Design review of the part shown in the three views and the two pictorial views. Dimensions are in mm from the part's minimum x, y and z. Round coordinates to 2 decimals unless told otherwise and drop trailing zeros. Loops run counter-clockwise (first coordinate to the right, second up) from the corner with the lowest first, then second, coordinate; pieces in that order, holes last. Notation, with made-up numbers: (9, 63) -> (35, 63) arc R26 cw to (35, 90) -> close; hole circle Ø10 at (60, 70). An arc over 180 degrees is marked (long way). Use a Markdown table: item, result. Add a question column.
1) Consider section B-B on x = 33. Give the boundary of the cut face in (y, z).
2) Consider section C-C on y = 2.4. Give the boundary of the cut face in (x, z), plus the area to 3 significant figures.
3) Wall thickness on probe 1 along Y at (x, z) = (79, 32); probe 2 along X at (y, z) = (0.9, 31.5); probe 3 along Z at (x, y) = (35, 3.2): over which ranges is each line inside the solid? List them lowest first.
4) Insertion check: pin 1 (1.6 mm diameter, centred on x = 32.5, y = 2.5, fed in from -Z); pin 2 (1.6 mm diameter, centred on x = 42.5, z = 34.5, fed in from -Y); pin 3 (3 mm diameter, centred on y = 4, z = 6.5, fed in from -X). Each pin has a flat end and moves straight along its axis. Give the tip position at first contact, or say it passes through.
5) Consider section A-A on z = 30. Give the boundary of the cut face in (x, y), plus the area to 3 significant figures.
6) Mouldability with a two-part tool opening along Y and no side actions: class the marked faces 1, 2 and 3 as released by +Y, released by -Y, zero draft, split by the parting line, or undercut.
7) Consider section D-D on z = 5. Give the boundary of the cut face in (x, y).
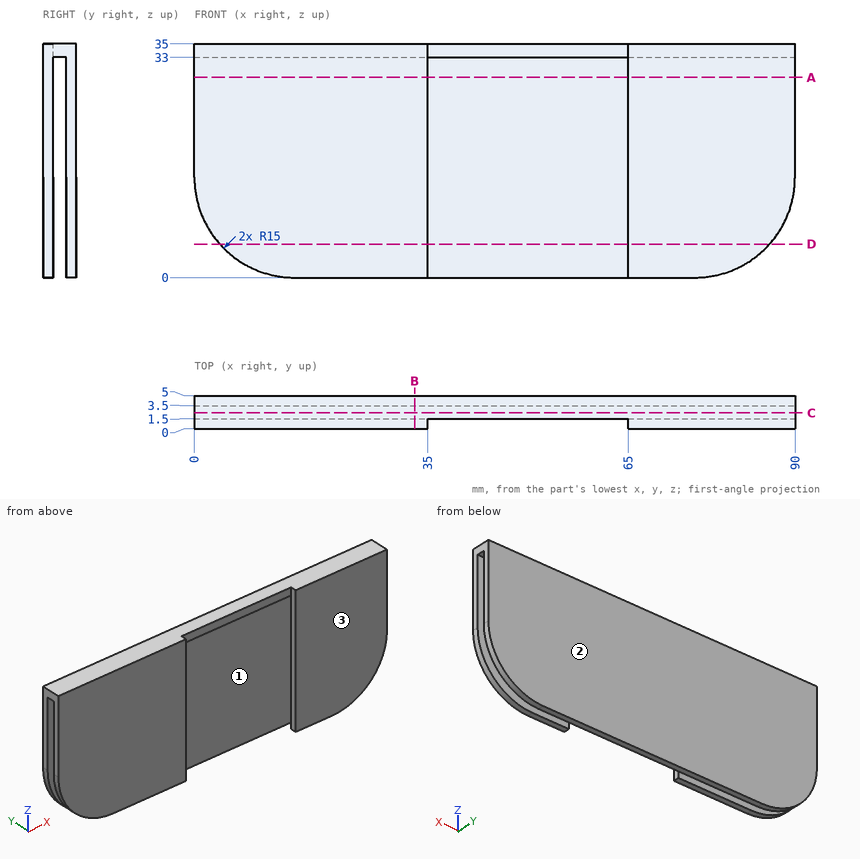
Result set:
| question | item | result |
|---|---|---|
| 1 | outline | (0, 0) -> (1.5, 0) -> (1.5, 33) -> (3.5, 33) -> (3.5, 0) -> (5, 0) -> (5, 35) -> (0, 35) -> close |
| 2 | outline | (0, 33) -> (90, 33) -> (90, 35) -> (0, 35) -> close |
| 2 | area | 180 mm2 |
| 3 | probe 1 | 0 to 1.5, 3.5 to 5 |
| 3 | probe 2 | 0 to 35, 65 to 90 |
| 3 | probe 3 | 33 to 35 |
| 4 | pin 1 | z = 33 |
| 4 | pin 2 | y = 1.5 |
| 4 | pin 3 | x = 1.73 |
| 5 | outline | (0, 0) -> (35, 0) -> (35, 1.5) -> (0, 1.5) -> close; (0, 3.5) -> (90, 3.5) -> (90, 5) -> (0, 5) -> close; (65, 0) -> (90, 0) -> (90, 1.5) -> (65, 1.5) -> close |
| 5 | area | 225 mm2 |
| 6 | face 1 | undercut |
| 6 | face 2 | released by +Y |
| 6 | face 3 | released by -Y |
| 7 | outline | (3.82, 0) -> (35, 0) -> (35, 1.5) -> (3.82, 1.5) -> close; (3.82, 3.5) -> (86.18, 3.5) -> (86.18, 5) -> (3.82, 5) -> close; (65, 0) -> (86.18, 0) -> (86.18, 1.5) -> (65, 1.5) -> close |
